from build123d import *

# Parameters (mm, degrees)
BOSS_EXTRUDE1_DEPTH = 2


with BuildPart() as part:
    # Sketch1 → Boss-Extrude1 (new body)
    with BuildSketch(Plane(origin=(0, 0, 0), x_dir=(1, 0, 0), z_dir=(0, 1, 0))):
        with BuildLine():
            Line((-20, 4), (-4, 4))
            ThreePointArc((-4, 4), (-1.878679656, 4.878679656), (-1, 7))
            Line((-1, 7), (-1, 28))
            ThreePointArc((-1, 28), (-0.121320344, 30.121320344), (2, 31))
            Line((2, 31), (4, 31))
            ThreePointArc((4, 31), (6.121320344, 30.121320344), (7, 28))
            Line((7, 28), (7, 7))
            ThreePointArc((7, 7), (7.878679656, 4.878679656), (10, 4))
            Line((10, 4), (24, 4))
            ThreePointArc((24, 4), (26.121320344, 4.878679656), (27, 7))
            Line((27, 7), (27, 28))
            ThreePointArc((27, 28), (27.878679656, 30.121320344), (30, 31))
            Line((30, 31), (32, 31))
            ThreePointArc((32, 31), (34.121320344, 30.121320344), (35, 28))
            Line((35, 28), (35, 7))
            ThreePointArc((35, 7), (35.878679656, 4.878679656), (38, 4))
            Line((38, 4), (59, 4))
            ThreePointArc((59, 4), (61.121320344, 3.121320344), (62, 1))
            Line((62, 1), (62, -1))
            ThreePointArc((62, -1), (61.121320344, -3.121320344), (59, -4))
            Line((59, -4), (-47, -4))
            ThreePointArc((-47, -4), (-49.121320344, -3.121320344), (-50, -1))
            Line((-50, -1), (-50, 1))
            ThreePointArc((-50, 1), (-49.121320344, 3.121320344), (-47, 4))
            Line((-47, 4), (-34, 4))
            ThreePointArc((-34, 4), (-31.878679656, 4.878679656), (-31, 7))
            Line((-31, 7), (-31, 28))
            ThreePointArc((-31, 28), (-30.121320344, 30.121320344), (-28, 31))
            Line((-28, 31), (-26, 31))
            ThreePointArc((-26, 31), (-23.878679656, 30.121320344), (-23, 28))
            Line((-23, 28), (-23, 7))
            ThreePointArc((-23, 7), (-22.121320344, 4.878679656), (-20, 4))
        make_face()
    extrude(amount=BOSS_EXTRUDE1_DEPTH)


solid = part.part
The model under review builds one solid part; all positions refer to its coordinate system, in mm. A direction names the side the tool comes from. Round coordinates to 2 decimals unless told otherwise and drop trailing zeros. Order: outer loops, then holes, each group sorted by start corner. A loop starts at its lowest first (then second) coordinate and runs counter-clockwise, first axis right, second up. Notation, with made-up numbers: (54, -29) - (98, -29) arc R24 cw to (98, 4) - close; hole circle Ø8 at (2.25, 78). An arc over 180 degrees is marked (long way). Use one line per item in the form item = value.
Q1. Clearance check with flat-ended pins moving along their axes: P1, Ø1, axis at x = -15.5, y = 0.5, coming from the -Z side; P2, Ø0.6, axis at y = 0.5, z = -13.5, coming from the +X side. State where each tip first meets the part, or that it passes through.
Response values:
P1 = -4
P2 = 35
Q2. Add section C-C on x = 14. Give the boundary of the cut face in (y, z).
Response values:
outline = (0, -4) - (2, -4) - (2, 4) - (0, 4) - close
Q3. Add section D-D on x = -3. Give the boundary of the cut face in (y, z), then the cut area to 3 significant figures.
Response values:
outline = (0, -4.17) - (2, -4.17) - (2, 4) - (0, 4) - close
area = 16.3 mm^2
Q4. To check wall thickness, follow line 1 (X direction, y = 0.75, z = -27.5); line 2 (Z direction, x = 13, y = 1.2); line 3 (X direction, y = 0.75, z = -2.5). State the ranges of each line that lie inside material, in increasing order.
Response values:
line_1 = -31 to -23, -1 to 7, 27 to 35
line_2 = -4 to 4
line_3 = -49.6 to 61.6
Q5. Tool access review of faces 1 (the cylindrical face through (-1.9, 0.99, -4.86)), 2 (the flat face through (35, 1, -18)), 3 (the flat face through (-41, 1, -4)): name each direction out of +Z, -Z, +X, -X, +Y, -Y from which nothing blocks a thin tool from reaching the whole face with its end or side.
Response values:
face_1 = -Z, +Y, -Y
face_2 = -Z, +X, +Y, -Y
face_3 = -Z, -X, +Y, -Y
Q6. Add section A-A on z = -15.5. Give the boundary of the cut face in (x, y), then the cut area to 3 significant figures.
Response values:
outline = (-31, 0) - (-23, 0) - (-23, 2) - (-31, 2) - close; (-1, 0) - (7, 0) - (7, 2) - (-1, 2) - close; (27, 0) - (35, 0) - (35, 2) - (27, 2) - close
area = 48.0 mm^2
Q7. Mouldability with a two-part tool opening along X and no side actions: class faces 4 (the cylindrical face through (-0.14, 0.99, -30.1)), 5 (the cylindrical face through (34.1, 0.99, -30.14)), 6 (the cylindrical face through (-49.1, 0.99, 3.14)) as pulls with the +X half, pulls with the -X half, needs draft (parallel to the pull), parting line crosses it, or undercut.
Response values:
face_4 = undercut
face_5 = pulls with the +X half
face_6 = pulls with the -X half
